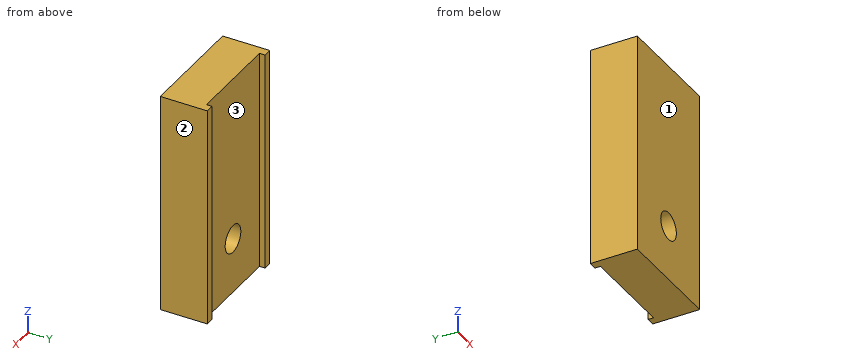
```python
from build123d import *

# Parameters (mm, degrees)
SKETCH1_W               = 25.4
SKETCH1_H               = 50.8
BOSS_EXTRUDE1_DEPTH     = 9.525
SKETCH2_W               = 1.905
SKETCH2_H               = 50.8
BOSS_EXTRUDE2_DEPTH     = 1.27
CUT_EXTRUDE1_DEPTH      = 30.952890094
CUT_EXTRUDE1_DEPTH_BACK = 30.952890094
SKETCH3_R               = 3.175


with BuildPart() as part:
    # Sketch1 → Boss-Extrude1 (new body)
    with BuildSketch(Plane(origin=(0, 0, 0), x_dir=(1, 0, 0), z_dir=(0, 1, 0))):
        Rectangle(SKETCH1_W, SKETCH1_H)
    extrude(amount=BOSS_EXTRUDE1_DEPTH)

    # Sketch2 → Boss-Extrude2 (add)
    with BuildSketch(Plane(origin=(0, 9.525, 0), x_dir=(1, 0, 0), z_dir=(0, 1, 0))):
        with Locations((-11.7475, 0)):
            Rectangle(SKETCH2_W, SKETCH2_H)
        with Locations((11.7475, 0)):
            Rectangle(SKETCH2_W, SKETCH2_H)
    extrude(amount=BOSS_EXTRUDE2_DEPTH)

    # Sketch3 → Cut-Extrude1 (cut, two sides: drawn at the far end of the back side and taken through both)
    with BuildSketch(Plane(origin=(0, 9.525, 0), x_dir=(1, 0, 0), z_dir=(0, 1, 0)).offset(-CUT_EXTRUDE1_DEPTH_BACK)):
        with Locations(Location((0, 12.7, 0), (0, 0, 270))):
            Circle(SKETCH3_R)
    extrude(amount=CUT_EXTRUDE1_DEPTH + CUT_EXTRUDE1_DEPTH_BACK, mode=Mode.SUBTRACT)


solid = part.part
```
Design review of the part built by this model. Coordinates are the model's own, in mm. Face numbers are marked on the shaded views. Coordinates: 2 decimals unless noted, no trailing zeros. Order: outer loops, then holes, each group sorted by start corner. A loop starts at its lowest first (then second) coordinate and runs counter-clockwise, first axis right, second up.
1) Clearance check with flat-ended pins moving along their axes: pin 1 (6 mm diameter, centred on x = -9, z = -4.5, fed in from -Y); pin 2 (6.5 mm diameter, centred on x = 1.5, z = -0.5, fed in from +Y) (3 decimals). State where each tip first meets the part, or that it passes through.
2) Mouldability with a two-part tool opening along X and no side actions: class the marked faces 1, 2 and 3 as +X half, -X half, draft (parallel to the pull), parting line (faces both ways), or undercut.
3) Take a section at D-D, the plane y = 9. Give the boundary of the cut face in (x, z) (3 decimals), and give its area (3 significant figures).
4) Wall thickness on line 1 along Z through (x, y) = (0, 6) (3 decimals); line 2 along X through (y, z) = (6.5, -12.7) (3 decimals); line 3 along X through (y, z) = (9.75, -2) (3 decimals): over which ranges is each line inside the solid? List them lowest first.
5) Take a section at C-C, the plane z = 17. Give the boundary of the cut face in (x, y) (3 decimals), and give its area (3 significant figures).
6) Take a section at B-B, the plane z = -12.7. Give the boundary of the cut face in (x, y) (3 decimals).
7) Take a section at A-A, the plane x = 0. Give the boundary of the cut face in (y, z) (3 decimals), and give its area (3 significant figures).
Returned:
1. pin 1: stops at y = 0
1. pin 2: stops at y = 9.525
2. face 1: draft
2. face 2: +X half
2. face 3: undercut
3. outline: (-12.7, -25.4) - (12.7, -25.4) - (12.7, 25.4) - (-12.7, 25.4) - close; hole circle Ø6.35 at (0, -12.7)
3. area: 1,260 mm2
4. line 1: z = -25.4 to -15.875, -9.525 to 25.4
4. line 2: x = -12.7 to -3.175, 3.175 to 12.7
4. line 3: x = -12.7 to -10.795, 10.795 to 12.7
5. outline: (-12.7, 0) - (12.7, 0) - (12.7, 10.795) - (10.795, 10.795) - (10.795, 9.525) - (-10.795, 9.525) - (-10.795, 10.795) - (-12.7, 10.795) - close
5. area: 247 mm2
6. outline: (-12.7, 0) - (-3.175, 0) - (-3.175, 9.525) - (-10.795, 9.525) - (-10.795, 10.795) - (-12.7, 10.795) - close; (3.175, 0) - (12.7, 0) - (12.7, 10.795) - (10.795, 10.795) - (10.795, 9.525) - (3.175, 9.525) - close
7. outline: (0, -25.4) - (9.525, -25.4) - (9.525, -15.875) - (0, -15.875) - close; (0, -9.525) - (9.525, -9.525) - (9.525, 25.4) - (0, 25.4) - close
7. area: 423 mm2
